Geometry check sheet. Reference: the model listing, model coordinates, mm. Face numbers are marked on the shaded views. Round coordinates to 2 decimals unless told otherwise and drop trailing zeros. Order: outer loops, then holes, each group sorted by start corner. A loop starts at its lowest first (then second) coordinate and runs counter-clockwise, first axis right, second up.
```python
from build123d import *

# Parameters (mm, degrees)
F0_W     = 45.5336533487
F0_H     = 64.6490454674
F1_DEPTH = 5
F2_R     = 2
F3_R     = 4.9143331214
F4_DEPTH = 1
F5_R     = 1.2295476181
F6_DEPTH = 5


with BuildPart() as f1:
    # F0 (on Top) → F1 (new body)
    with BuildSketch(Plane.XY):
        with Locations((22.7668266743, 32.3245227337)):
            Rectangle(F0_W, F0_H)
    extrude(amount=F1_DEPTH)

    # F2
    f2_edges = [f1.edges().sort_by_distance(p)[0] for p in [
        (0, 64.649045, 2.5),
        (0, 0, 2.5),
        (0, 32.324523, 0),
        (0, 32.324523, 5),
        (45.533653, 0, 2.5),
        (45.533653, 64.649045, 2.5),
        (45.533653, 32.324523, 0),
        (45.533653, 32.324523, 5),
    ]]
    fillet(f2_edges, radius=F2_R)

    # F3 (on face) → F4 (cut)
    with BuildSketch(Plane.XY.offset(5)):
        with Locations((23.9143331214, 7.975962013)):
            Circle(F3_R)
    extrude(amount=-F4_DEPTH, mode=Mode.SUBTRACT)

    # F5 (on face) → F6 (cut)
    with BuildSketch(Plane(origin=(0, 64.6490454674, 0), x_dir=(-1, 0, 0), z_dir=(0, 1, 0))):
        with Locations((-40.4135324061, 2.5)):
            Circle(F5_R)
    extrude(amount=-F6_DEPTH, mode=Mode.SUBTRACT)


solid = f1.part
```
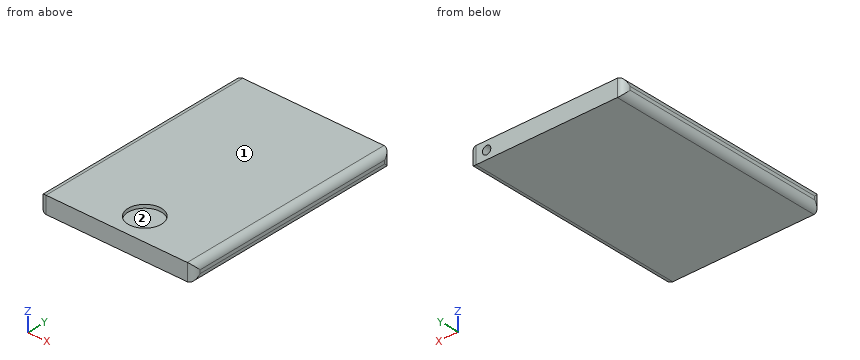
(1) Draft check along X on the marked faces 1 and 2. Enter one of: released by +X, released by -X, zero draft, split by the parting line, or undercut.
Returned:
face 1: zero draft
face 2: undercut
(2) Material ranges on line 1 (Z direction, x = 21, y = 8); line 2 (X direction, y = 42, z = 3.55); line 3 (Y direction, x = 20, z = 4.4), recorded low to high.
Returned:
line 1: z = 0 to 4
line 2: x = 0.08 to 45.46
line 3: y = 0 to 5, 10.95 to 64.65
(3) Depth check by flat-ended pin: P1, Ø8, axis at x = 23.91, y = 7.98, coming from the +Z side. Enter the tip coordinate at first touch or a pass-through.
Returned:
P1: stops at z = 4
(4) Sectioned sample at A-A, the plane y = 54.5. Record the cut outline in (x, z).
Returned:
outline: (0, 2) arc R2 ccw to (2, 0) - (43.53, 0) arc R2 ccw to (45.53, 2) - (45.53, 3) arc R2 ccw to (43.53, 5) - (2, 5) arc R2 ccw to (0, 3) - close
